For this review, take the finished solid that the model builds, in its own axes (mm). Coordinates: 2 decimals unless noted, no trailing zeros. Write each loop counter-clockwise with the first axis right and the second up, starting at its lowest first coordinate (ties: lowest second). Pieces come first, ordered by that corner, then holes. Notation, with made-up numbers: M 37.25,14 L 54.25,14 A27 cw 54.25,33 Z; hole C -34,33.5 d11. An arc over 180 degrees is marked long. One line per question, with ' | ' between items.
from build123d import *

# Parameters (mm, degrees)
F1_DEPTH = 15
F3_DEPTH = 60
F4_SIZE  = 3
F5_R     = 5


with BuildPart() as f1:
    # F0 (on Top) → F1 (new body)
    with BuildSketch(Plane.XY):
        Polygon((-84.375, 42.2187384345), (-78.75, 45.4663336987), (-61.4294919243, 55.4663336987), (-63.9294919243, 59.7964607176), (-72.5897459622, 54.7964607176), (-75.7147459622, 60.2091194913), (-84.375, 55.2091194913), (-81.25, 49.7964607176), (-86.875, 46.5488654534), align=None)
        Polygon((-61.4294919243, 55.4663336987), (-57.0993649054, 57.9663336987), (-59.5993649054, 62.2964607176), (-63.9294919243, 59.7964607176), align=None)
        Polygon((-91.7403810568, 37.9663336987), (-84.375, 42.2187384345), (-86.875, 46.5488654534), (-94.2403810568, 42.2964607176), align=None)
        Polygon((-84.375, 55.2091194913), (-75.7147459622, 60.2091194913), (-85.7147459622, 77.5296275669), (-87.793790014, 76.329290924), (-94.375, 72.5296275669), align=None)
        Polygon((-87.793790014, 76.329290924), (-85.7147459622, 77.5296275669), (-88.8397459622, 82.9422863406), (-75.8493649054, 90.4422863406), (-78.3493115936, 94.7723526968), (-100, 82.2724133595), (-105.625, 79.0248180953), (-103.125, 74.6946910764), (-97.5, 77.9422863406), (-94.375, 72.5296275669), align=None)
        Polygon((-110.4903810568, 70.4422863406), (-103.125, 74.6946910764), (-105.625, 79.0248180953), (-112.9903810568, 74.7724133595), align=None)
    extrude(amount=F1_DEPTH)

    # F2 (on face) → F3 (cut)
    with BuildSketch(Plane(origin=(-39.375, 68.199500548, 0), x_dir=(0.8660254038, 0.5, 0), z_dir=(0.5, -0.8660254038, 0))):
        with BuildLine():
            ThreePointArc((-52.7163336987, 7.5), (-55.4663336987, 10.25), (-58.2163336987, 7.5))
            Line((-58.2163336987, 7.5), (-55.4663336987, 7.5))
            Line((-55.4663336987, 7.5), (-52.7163336987, 7.5))
        make_face()
        with BuildLine():
            Line((-55.4663336987, 7.5), (-58.2163336987, 7.5))
            ThreePointArc((-58.2163336987, 7.5), (-55.4663336987, 4.75), (-52.7163336987, 7.5))
            Line((-52.7163336987, 7.5), (-55.4663336987, 7.5))
        make_face()
        with BuildLine():
            ThreePointArc((-22.8953336987, 7.5), (-25.6453336987, 10.25), (-28.3953336987, 7.5))
            ThreePointArc((-28.3953336987, 7.5), (-25.6453336987, 4.75), (-22.8953336987, 7.5))
        make_face()
    extrude(amount=-F3_DEPTH, mode=Mode.SUBTRACT)

    # F4
    f4_edges = [f1.edges().sort_by_distance(p)[0] for p in [
        (-89.375, 63.869374, 15),
        (-80.714746, 68.869374, 15),
        (-89.375, 63.869374, 0),
        (-80.714746, 68.869374, 0),
    ]]
    chamfer(f4_edges, length=F4_SIZE)

    # F5
    f5_edges = [f1.edges().sort_by_distance(p)[0] for p in [
        (-92.990381, 40.131397, 0),
        (-111.740381, 72.60735, 0),
        (-111.740381, 72.60735, 15),
        (-92.990381, 40.131397, 15),
        (-58.349365, 60.131397, 15),
        (-58.349365, 60.131397, 0),
        (-77.099338, 92.60732, 15),
        (-77.099338, 92.60732, 0),
    ]]
    fillet(f5_edges, radius=F5_R)


solid = f1.part
1) We need section B-B on y = 63. State the section outline as (x, z) points, then the cut area to 3 significant figures.
Responses:
outline: M -88.87,3 L -85.41,0 L -80.79,0 L -77.33,3 L -77.33,12 L -80.79,15 L -85.41,15 L -88.87,12 Z | area: 152 mm^2
2) The part is to be moulded in two halves that separate along X. For faces 1 (the cylindrical face through (-110.421, 73.329, 13.574)), 2 (the flat face through (-58.33, 60.1, 7.46)), 3 (the cylindrical face through (-90.914, 41.29, 6.674)), 4 (the flat face through (-85, 66, 0)), say which applies: +X half, -X half, draft (parallel to the pull), parting line (faces both ways), or undercut.
Responses:
face 1: -X half | face 2: +X half | face 3: undercut | face 4: draft
3) We need section D-D on x = -67.5. State the section outline as (y, z) points, then the cut area to 3 significant figures.
Responses:
outline: M 51.96,0 L 57.74,0 L 57.74,15 L 51.96,15 Z | area: 86.6 mm^2
4) We need section C-C on z = 9. State how many separate pieces and enclosed holes the cut face has, then the cut area to 3 significant figures.
Responses:
separate pieces: 5 | enclosed holes: 0 | area: 633 mm^2
5) To check wall thickness, follow line 1 along X through (y, z) = (58, 7.5); line 2 along Y through (x, z) = (-79, 4.25); line 3 along X through (y, z) = (77.5, 13.5). State the ranges of each line that lie inside material, in increasing order. Write a range as [from, to].
Responses:
line 1: [-85.99, -74.44], [-67.04, -66.27], [-59.92, -57.12] | line 2: [45.32, 65.9], [88.62, 94.4] | line 3: [-108.27, -98.27], [-95.51, -87.43]
6) Insertion check: pin 1 Ø8 at (x, z) = (-73.5, 12.5) entering from +Y; pin 2 Ø8 at (x, z) = (-84.5, 12.5) entering from -Y; pin 3 Ø5 at (y, z) = (82.5, 11.5) entering from +X. Each pin has a flat end and moves straight along its axis. Give the tip position at first contact, or say it passes through.
Responses:
pin 1: y = 92.64 | pin 2: y = 39.84 | pin 3: x = -85.28
